from build123d import *

# Parameters (mm, degrees)
SKETCH2_R           = 0.75
BOSS_EXTRUDE1_DEPTH = 7.5
CUT_EXTRUDE1_DEPTH  = 5
SKETCH4_R           = 2.25
BOSS_EXTRUDE2_DEPTH = 5


with BuildPart() as part:
    # Sketch2 → Boss-Extrude1 (new body)
    with BuildSketch(Plane(origin=(0, 0, 0), x_dir=(1, 0, 0), z_dir=(0, 1, 0))):
        with BuildLine():
            Line((-1.245487365, 94.918772563), (-1.245487365, 4.918772563))
            ThreePointArc((-1.245487365, 4.918772563), (6.254512635, -2.581227437), (13.754512635, 4.918772563))
            Line((13.754512635, 4.918772563), (13.754512635, 94.918772563))
            ThreePointArc((13.754512635, 94.918772563), (6.254512635, 102.418772563), (-1.245487365, 94.918772563))
        make_face()
        with Locations(Location((4.754512635, 4.918772563, 0), (0, 0, 270))):
            Circle(SKETCH2_R, mode=Mode.SUBTRACT)
        with Locations(Location((7.754512635, 4.918772563, 0), (0, 0, 270))):
            Circle(SKETCH2_R, mode=Mode.SUBTRACT)
    extrude(amount=BOSS_EXTRUDE1_DEPTH)

    # Sketch3 → Cut-Extrude1 (cut)
    with BuildSketch(Plane.XZ):
        with BuildLine():
            Line((11.254512635, -4.918772563), (11.254512635, -44.918772563))
            ThreePointArc((11.254512635, -44.918772563), (6.254512635, -49.918772563), (1.254512635, -44.918772563))
            Line((1.254512635, -44.918772563), (1.254512635, -4.918772563))
            ThreePointArc((1.254512635, -4.918772563), (6.254512635, 0.081227437), (11.254512635, -4.918772563))
        make_face()
    extrude(amount=-CUT_EXTRUDE1_DEPTH, mode=Mode.SUBTRACT)

    # Sketch4 → Boss-Extrude2 (add)
    with BuildSketch(Plane(origin=(0, 7.5, 0), x_dir=(1, 0, 0), z_dir=(0, 1, 0))):
        with Locations(Location((6.254512635, 94.918772563, 0), (0, 0, 270))):
            Circle(SKETCH4_R)
    extrude(amount=BOSS_EXTRUDE2_DEPTH)


solid = part.part
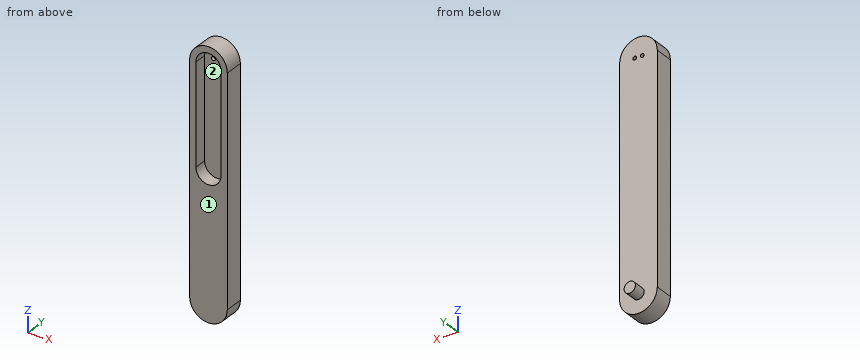
For this review, take the finished solid that the model builds, in its own axes (mm). Face numbers are marked on the shaded views. A direction names the side the tool comes from. Round coordinates to 2 decimals unless told otherwise and drop trailing zeros. Loops run counter-clockwise (first coordinate to the right, second up) from the corner with the lowest first, then second, coordinate; pieces in that order, holes last. Notation, with made-up numbers: (23.25, -34.75) - (61.25, -34.75) arc R13 ccw to (61.25, -26.75) - close; hole circle Ø1 at (-37, 24.5). An arc over 180 degrees is marked (long way). One line per item, written item: value. Start each with the question number.
Item 1: For L1, parallel to X at y = 1, z = -25.5; L2, parallel to Y at x = 0.25, z = -45; L3, parallel to Y at x = 9.5, z = -41, list the stretches that pass through material, from the lowest coordinate up.
Item 2: For the marked faces 1 and 2, list the 3-axis set-ups (+Z, -Z, +X, -X, +Y, -Y) from which the entire face can be reached by the end or side of a thin tool; tool diameter is ignored.
Item 3: Take a section at B-B (z = -39). Give the boundary of the cut face in (x, y).
Item 4: Take a section at D-D (z = -72). Give the boundary of the cut face in (x, y).
Item 5: Take a section at C-C (x = 2.75). Give the boundary of the cut face in (y, z), plus the area to 3 significant figures.
Item 6: Clearance check with flat-ended pins moving along their axes: pin 1 Ø1 at (x, z) = (2.5, -42.5) entering from +Y; pin 2 Ø4 at (x, y) = (2.5, 7) entering from -Z; pin 3 Ø0.9 at (x, z) = (4.75, -4.92) entering from +Y; pin 4 Ø2 at (x, z) = (7.75, -4.92) entering from -Y. State where each tip first meets the part, or that it passes through.
Item 7: Take a section at A-A (y = 1). Give the boundary of the cut face in (x, z), plus the area to 3 significant figures.
Answer below:
1. L1: x = -1.25 to 1.25, 11.25 to 13.75
1. L2: y = 0 to 7.5
1. L3: y = 5 to 7.5
2. face 1: +Z, -Z, +X, -X, -Y
2. face 2: -Y
3. outline: (-1.25, 0) - (1.25, 0) - (1.25, 5) - (11.25, 5) - (11.25, 0) - (13.75, 0) - (13.75, 7.5) - (-1.25, 7.5) - close
4. outline: (-1.25, 0) - (13.75, 0) - (13.75, 7.5) - (-1.25, 7.5) - close
5. outline: (0, -101.55) - (7.5, -101.55) - (7.5, 1.71) - (0, 1.71) - (0, -1.35) - (5, -1.35) - (5, -48.49) - (0, -48.49) - close
5. area: 539 mm2
6. pin 1: stops at y = 7.5
6. pin 2: stops at z = -102.21
6. pin 3: passes through
6. pin 4: stops at y = 5
7. outline: (-1.25, -94.92) arc R7.5 ccw to (13.75, -94.92) - (13.75, -4.92) arc R7.5 ccw to (-1.25, -4.92) - close; hole (1.25, -44.92) arc R5 ccw to (11.25, -44.92) - (11.25, -4.92) arc R5 ccw to (1.25, -4.92) - close
7. area: 1,050 mm2
